Read the model definition and answer for the solid it produces. Units are mm, in the model's axes. Face numbers are marked on the shaded views. Give positions to 0.01 mm unless a question says otherwise; leave off trailing zeros. Write each loop counter-clockwise with the first axis right and the second up, starting at its lowest first coordinate (ties: lowest second). Pieces come first, ordered by that corner, then holes. Notation, with made-up numbers: (-2.75, -11) -> (5.25, -11) arc R19 ccw to (5.25, -7) -> close; hole circle Ø1 at (36.25, -30.75). An arc over 180 degrees is marked (long way). Put each result on its own line as item: value. Start each with the question number.
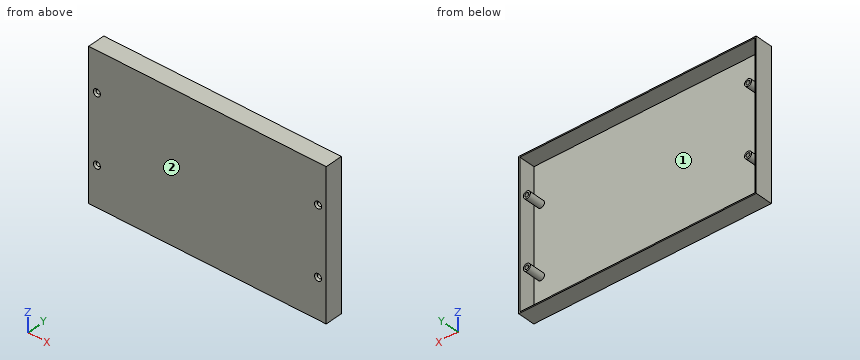
from build123d import *

# Parameters (mm, degrees)
SKETCH_W         = 204
SKETCH_H         = 126
PAD_DEPTH        = 15
SKETCH001_W      = 202
SKETCH001_H      = 124
POCKET_DEPTH     = 14
SKETCH002_R      = 3
PAD001_DEPTH     = 15
HOLE_D           = 3.4
HOLE_DEPTH       = 25
HOLE_CSINK_D     = 6.1
HOLE_CSINK_ANGLE = 90


with BuildPart() as part:
    # Sketch → Pad (new body)
    with BuildSketch(Plane.XZ):
        Rectangle(SKETCH_W, SKETCH_H)
    extrude(amount=-PAD_DEPTH)

    # Sketch001 (on Face6 of Pad) → Pocket (cut)
    with BuildSketch(Plane(origin=(0, 15, 0), x_dir=(1, 0, 0), z_dir=(0, 1, 0))):
        Rectangle(SKETCH001_W, SKETCH001_H)
    extrude(amount=-POCKET_DEPTH, mode=Mode.SUBTRACT)

    # Sketch002 (on Face4 of Pocket) → Pad001 (join)
    with BuildSketch(Plane.XZ):
        with Locations((-95, 29)):
            Circle(SKETCH002_R)
        with Locations((95, 29)):
            Circle(SKETCH002_R)
        with Locations((95, -29)):
            Circle(SKETCH002_R)
        with Locations((-95, -29)):
            Circle(SKETCH002_R)
    extrude(amount=-PAD001_DEPTH)

    # Hole
    with Locations(Plane.XZ):
        with Locations((-95, 29), (95, 29), (95, -29), (-95, -29)):
            CounterSinkHole(HOLE_D / 2, HOLE_CSINK_D / 2, depth=HOLE_DEPTH, counter_sink_angle=HOLE_CSINK_ANGLE)


solid = part.part
1) A cutting plane is placed at C-C on x = -48. Give the vertices of the cut face in (y, z), and give its area (3 significant figures).
2) Straight lines are drawn through the part: line 1 (Z direction, x = 95, y = 7.5); line 2 (Z direction, x = -35, y = 5.5); line 3 (X direction, y = 2.25, z = -40.5). For each, find the intervals that lie inside material, in ascending order. Write a range as [from, to].
3) Each of these flat-tipped pins is pushed along its axis until it touches: pin 1 Ø6 at (x, z) = (-64, -49) entering from +Y; pin 2 Ø5.5 at (x, z) = (-95, -29) entering from -Y; pin 3 Ø5.5 at (x, z) = (95, -29) entering from +Y; pin 4 Ø4 at (x, z) = (95, 29) entering from -Y. Where does it stop, or does it pass through?
4) For a pull along Z with two mould halves and no side action, classify the marked faces 1 and 2 as pulls with the +Z half, pulls with the -Z half, needs draft (parallel to the pull), parting line crosses it, or undercut.
5) A cutting plane is placed at A-A on y = 7.5. State how many separate pieces and enclosed holes the cut face has, and give its area (3 significant figures).
6) A cutting plane is placed at B-B on z = 17.5. Give the vertices of the cut face in (x, y).
Results found:
1. outline: (0, -63) -> (15, -63) -> (15, -62) -> (1, -62) -> (1, 62) -> (15, 62) -> (15, 63) -> (0, 63) -> close
1. area: 154 mm²
2. line 1: z = [-63, -62], [-32, -30.7], [-27.3, -26], [26, 27.3], [30.7, 32], [62, 63]
2. line 2: z = [-63, -62], [62, 63]
2. line 3: x = [-102, -101], [101, 102]
3. pin 1: stops at y = 1
3. pin 2: stops at y = 0.3
3. pin 3: stops at y = 15
3. pin 4: stops at y = 1.05
4. face 1: undercut
4. face 2: needs draft
5. separate pieces: 5
5. enclosed holes: 5
5. area: 733 mm²
6. outline: (-102, 0) -> (102, 0) -> (102, 15) -> (101, 15) -> (101, 1) -> (-101, 1) -> (-101, 15) -> (-102, 15) -> close
